For this review, take the finished solid that the model builds, in its own axes (mm). Face numbers are marked on the shaded views. Round coordinates to 2 decimals unless told otherwise and drop trailing zeros. Order: outer loops, then holes, each group sorted by start corner. A loop starts at its lowest first (then second) coordinate and runs counter-clockwise, first axis right, second up. Notation, with made-up numbers: (-4.75, 21) - (28.25, 21) arc R14 ccw to (28.25, 41) - close; hole circle Ø1 at (75, 46.5). An arc over 180 degrees is marked (long way). One line per item, written item: value.
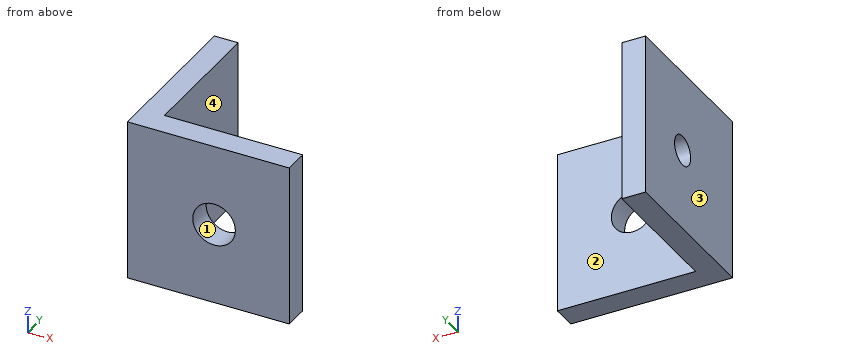
Autodesk Inventor part; units mm, degrees
ref_plane "YZ Plane" through (0, 0, 0) normal (1, 0, 0) x (0, 1, 0)
ref_plane "XZ Plane" through (0, 0, 0) normal (0, 1, 0) x (-1, 0, 0)
ref_plane "XY Plane" through (0, 0, 0) normal (0, 0, 1) x (1, 0, 0)
sketch "Sketch1" plane through (0, 0, 0) normal (1, 0, 0) x (0, 1, 0)
  circle A0 centre (77.4226, -114.2734) radius 1.75
  line L0 (66.4726, -104.7484) -> (66.4726, -123.7984)
  line L1 (66.4726, -104.7484) -> (85.5226, -104.7484)
  line L2 (85.5226, -123.7984) -> (85.5226, -104.7484)
  line L3 (66.4726, -123.7984) -> (85.5226, -123.7984)
  point P0 (0, 0)
extrude "Extrusion1" add sketch "Sketch1" along normal blind 2.794
sketch "Sketch3" plane through (2.794, 0, 0) normal (1, 0, 0) x (0, 0, -1)
  line L0 (104.7484, 66.4726) -> (123.7984, 66.4726)
  line L1 (104.7484, 85.5226) -> (104.7484, 66.4726)
  line L2 (104.7484, 66.4726) -> (104.7484, 69.3936)
  line L3 (104.7484, 66.4726) -> (107.6694, 66.4726) construction
  line L4 (123.7984, 66.4726) -> (123.7984, 85.5226)
  line L5 (123.7984, 66.4726) -> (123.7984, 69.3936)
  line L6 (123.7984, 66.4726) -> (126.7194, 66.4726) construction
  line L7 (123.7984, 69.3936) -> (104.7484, 69.3936)
  point P0 (0, 0)
  dimension "d2" = 2.921
  dimension "d3" = 90
  dimension "d4" = 2.921
  dimension "d5" = 90
extrude "Extrusion2" add sketch "Sketch3" along normal blind 16.256
sketch "Sketch4" plane through (2.794, 69.3936, -104.7484) normal (0, 1, 0) x (1, 0, 0)
  line L0 (16.256, 19.05) -> (16.256, 0) construction
  line L1 (16.256, 0) -> (16.256, 19.05) construction
  line L2 (16.256, 9.525) -> (7.406, 9.525) construction
  circle A0 centre (7.406, 9.525) radius 2.5
  point P0 (-2.794, -104.7484)
  dimension "d8" = 8.85
  dimension "d9" = 5
extrude "Extrusion3" cut sketch "Sketch4" against normal blind 16.256
Item 1: Take a section at C-C (z = -109.5). Write out the cut boundary in (x, y).
Returned:
outline: (0, 66.47) - (19.05, 66.47) - (19.05, 69.39) - (2.79, 69.39) - (2.79, 85.52) - (0, 85.52) - close
Item 2: Wall thickness on line 1 (Z direction, x = 1.5, y = 77.5); line 2 (Y direction, x = 9.5, z = -118.75); line 3 (X direction, y = 72.75, z = -109.75): over which ranges is each line inside the solid? List them lowest first.
Returned:
line 1: -123.8 to -116.02, -112.53 to -104.75
line 2: 66.47 to 69.39
line 3: 0 to 2.79
Item 3: Take a section at D-D (y = 72.5). Write out the cut boundary in (x, z), plus the area to 3 significant figures.
Returned:
outline: (0, -123.8) - (2.79, -123.8) - (2.79, -104.75) - (0, -104.75) - close
area: 53.2 mm^2
Item 4: Take a section at A-A (x = 10.2). Write out the cut boundary in (y, z), plus the area to 3 significant figures.
Returned:
outline: (66.47, -123.8) - (69.39, -123.8) - (69.39, -116.77) - (66.47, -116.77) - close; (66.47, -111.77) - (69.39, -111.77) - (69.39, -104.75) - (66.47, -104.75) - close
area: 41.0 mm^2
Item 5: For P1, Ø1.5, axis at x = 4.5, z = -113.5, coming from the +Y side; P2, Ø5, axis at x = 4.5, y = 70, coming from the +Z side; P3, Ø1.5, axis at y = 81, z = -108.5, coming from the +X side, all flat-tipped, find the tip position at first contact; note any pin that passes through.
Returned:
P1: y = 69.39
P2: z = -104.75
P3: x = 2.79
Item 6: Take a section at B-B (y = 76). Write out the cut boundary in (x, z).
Returned:
outline: (0, -123.8) - (2.79, -123.8) - (2.79, -115.29) - (0, -115.29) - close; (0, -113.25) - (2.79, -113.25) - (2.79, -104.75) - (0, -104.75) - close
Item 7: The part is to be moulded in two halves that separate along X. For the marked faces 1, 2, 3 and 4, say which applies: +X half, -X half, draft (parallel to the pull), parting line (faces both ways), or undercut.
Returned:
face 1: undercut
face 2: draft
face 3: -X half
face 4: +X half
